```python
from build123d import *

# Parameters (mm, degrees)
F0_R          = 31.75
F1_DEPTH      = 17.78
F2_T          = -2.54
F3_W          = 1.858536154
F3_H          = 11.058293283
F4_DEPTH      = 10.16
F5_W          = 5.9044365771
F5_H          = 11.058293283
F6_DEPTH      = 0.762
F7_W          = 58.5439018905
F7_H          = 1.300974749
F8_DEPTH      = 43.434
F8_DEPTH_BACK = 25.4
F10_START     = 30.607
F9_W          = 2.780330833
F9_H          = 1.4108410105
F10_DEPTH     = 3.683


with BuildPart() as f1:
    # F0 (on Top) → F1 (new body)
    with BuildSketch(Plane.XY):
        Circle(F0_R)
    extrude(amount=F1_DEPTH)

    # F2
    f2_openings = [f1.faces().sort_by_distance(p)[0] for p in [
        (0, 0, 17.78),
    ]]
    offset(amount=F2_T, openings=f2_openings)

    # F3 (on face) → F4 (join)
    with BuildSketch(Plane.XY.offset(2.54)):
        with Locations((-6.6907317378, 5.5291466415)):
            Rectangle(F3_W, F3_H)
        with Locations((6.6907317378, 5.5291466415)):
            Rectangle(F3_W, F3_H)
    extrude(amount=F4_DEPTH)

    # F5 (on face) → F6 (join)
    with BuildSketch(Plane.XY.offset(12.7)):
        with Locations((-8.7136819493, 5.5291466415)):
            Rectangle(F5_W, F5_H)
        with Locations((8.7136819493, 5.5291466415)):
            Rectangle(F5_W, F5_H)
    extrude(amount=F6_DEPTH)

    # F7 (on Right) → F8 (cut, two sides)
    with BuildSketch(Plane.YZ) as f8_sk:
        with Locations((0.6504878402, 14.8682934232)):
            Rectangle(F7_W, F7_H)
    extrude(amount=F8_DEPTH, mode=Mode.SUBTRACT)
    extrude(f8_sk.sketch, amount=-F8_DEPTH_BACK, mode=Mode.SUBTRACT)

    # F9 (on Right) → F10 (cut)
    with BuildSketch(Plane.YZ.offset(F10_START)):
        with Locations((-1.3901654165, 15.8451446332)):
            Rectangle(F9_W, F9_H)
        with Locations((1.3901654165, 15.8451446332)):
            Rectangle(F9_W, F9_H)
    extrude(amount=F10_DEPTH, mode=Mode.SUBTRACT)


solid = f1.part
```
Input: part model. Units: mm. Frame: model coordinates. A direction names the side the tool comes from. Give positions to 0.01 mm unless a question says otherwise; leave off trailing zeros. Order: outer loops, then holes, each group sorted by start corner. A loop starts at its lowest first (then second) coordinate and runs counter-clockwise, first axis right, second up. Notation, with made-up numbers: M 8,74.5 L 45,74.5 A6 cw 45,81.5 Z; hole C 21,89.25 d8. An arc over 180 degrees is marked long. One line per question, with ' | ' between items. Start each with the question number.
1. Section query D-D (x = 0). Return the cut outline in (y, z).
2. First-contact query: pin 1 Ø4 at (x, z) = (-4.5, 8.5) entering from -Y; pin 2 Ø0.5 at (y, z) = (1, 16) entering from +X; pin 3 Ø1.8 at (x, y) = (-8, 4.5) entering from +Z. Flat tips, straight axial feed; report the tip coordinate or a pass-through.
3. Material intervals for probe 1 along Y at (x, z) = (0, 13); probe 2 along Z at (x, y) = (-11, 4.5); probe 3 along Z at (x, y) = (21.5, 20), sorted ascending. Write a range as [from, to].
4. Section query C-C (y = 13). Return the cut outline in (x, z).
5. Pull-direction query (Z, two-part tool) for faces 4 (the face through (10, 6, 12.7)), 5 (the face through (-7, 11.058, 9)), 6 (the face through (9, 6, 13.462)); classes: released by +Z, released by -Z, zero draft, split by the parting line, or undercut.
6. Section query B-B (x = -18.5). Return the cut outline in (y, z), and give its area (3 significant figures).
7. Section query A-A (z = 6.5). Return the cut outline in (x, y).
8. Access query for faces 1 (the face through (0, 0, 0)), 2 (the face through (5.761, 5, 8)), 3 (the face through (-7.62, 5, 8)). Directions: +Z, -Z, +X, -X, +Y, -Y. A direction counts if a zero-diameter tool reaches every point of the face in a straight line with its end or side. Return the directions, or none.
Here are the results:
1) outline: M -31.75,0 L 31.75,0 L 31.75,17.78 L 29.21,17.78 L 29.21,15.52 L 29.92,15.52 L 29.92,14.22 L 29.21,14.22 L 29.21,2.54 L -29.21,2.54 L -29.21,17.78 L -31.75,17.78 Z
2) pin 1: y = -31.65 | pin 2: x = 30.61 | pin 3: z = 13.46
3) probe 1: [-31.75, -29.21], [29.21, 31.75] | probe 2: [0, 2.54], [12.7, 13.46] | probe 3: [0, 14.22], [15.52, 17.78]
4) outline: M -28.97,0 L 28.97,0 L 28.97,14.22 L 26.16,14.22 L 26.16,2.54 L -26.16,2.54 L -26.16,17.78 L -28.97,17.78 Z; M 26.16,15.52 L 28.97,15.52 L 28.97,17.78 L 26.16,17.78 Z
5) face 4: undercut | face 5: zero draft | face 6: released by +Z
6) outline: M -25.8,0 L 25.8,0 L 25.8,14.22 L 22.6,14.22 L 22.6,2.54 L -22.6,2.54 L -22.6,14.22 L -25.8,14.22 Z; M -25.8,15.52 L -22.6,15.52 L -22.6,17.78 L -25.8,17.78 Z; M 22.6,15.52 L 25.8,15.52 L 25.8,17.78 L 22.6,17.78 Z | area: 220 mm²
7) outline: C 0,0 d63.5; M -7.62,0 L -5.76,0 L -5.76,11.06 L -7.62,11.06 Z; M 5.76,0 L 7.62,0 L 7.62,11.06 L 5.76,11.06 Z; hole C 0,0 d58.42
8) face 1: -Z, +X, -X, +Y, -Y | face 2: +Z | face 3: none
